The listing builds one solid part. Answer for the finished solid, in the listing's coordinates (mm). A direction names the side the tool comes from. Coordinates: 2 decimals unless noted, no trailing zeros. Order: outer loops, then holes, each group sorted by start corner. A loop starts at its lowest first (then second) coordinate and runs counter-clockwise, first axis right, second up. Notation, with made-up numbers: (47, 76) -> (86, 76) arc R28 ccw to (86, 99) -> close; hole circle Ø9 at (-13, 12.25). An arc over 180 degrees is marked (long way). Return JSON: item names as keys, results as strings.
from build123d import *

# Parameters (mm, degrees)
SKETCH1_R               = 5.15
BOSS_EXTRUDE1_DEPTH     = 10.3
SKETCH2_R               = 1
CUT_EXTRUDE1_DEPTH      = 10
CUT_EXTRUDE1_DEPTH_BACK = 10
SKETCH3_W               = 4.05
SKETCH3_H               = 4.05
CUT_EXTRUDE2_DEPTH      = 5


with BuildPart() as part:
    # Sketch1 → Boss-Extrude1 (new body)
    with BuildSketch(Plane.XY):
        Circle(SKETCH1_R)
    extrude(amount=BOSS_EXTRUDE1_DEPTH)

    # Sketch2 → Cut-Extrude1 (cut, two sides)
    with BuildSketch(Plane(origin=(0, 0, 0), x_dir=(1, 0, 0), z_dir=(0, 1, 0))) as cut_extrude1_sk:
        with Locations((0, -7.5)):
            Circle(SKETCH2_R)
    extrude(amount=CUT_EXTRUDE1_DEPTH, mode=Mode.SUBTRACT)
    extrude(cut_extrude1_sk.sketch, amount=-CUT_EXTRUDE1_DEPTH_BACK, mode=Mode.SUBTRACT)

    # Sketch3 → Cut-Extrude2 (cut)
    with BuildSketch(Plane(origin=(0, 0, 0), x_dir=(-1, 0, 0), z_dir=(0, 0, -1))):
        Rectangle(SKETCH3_W, SKETCH3_H)
    extrude(amount=-CUT_EXTRUDE2_DEPTH, mode=Mode.SUBTRACT)


solid = part.part
1. The part is cut by section A-A on x = 0. Give the vertices of the cut face in (y, z) (3 decimals), and give its area (3 significant figures).
Answer block:
{"outline": "(-5.15, 0) -> (-2.025, 0) -> (-2.025, 5) -> (2.025, 5) -> (2.025, 0) -> (5.15, 0) -> (5.15, 6.5) -> (-5.15, 6.5) -> close; (-5.15, 8.5) -> (5.15, 8.5) -> (5.15, 10.3) -> (-5.15, 10.3) -> close", "area": "65.2 mm2"}
2. The part is cut by section C-C on y = 0.75. Give the vertices of the cut face in (x, z) (3 decimals).
Answer block:
{"outline": "(-5.095, 0) -> (-2.025, 0) -> (-2.025, 5) -> (2.025, 5) -> (2.025, 0) -> (5.095, 0) -> (5.095, 10.3) -> (-5.095, 10.3) -> close; hole circle Ø2 at (0, 7.5)"}
3. Consider line 1 (Z direction, x = 0, y = -3.95); line 2 (Z direction, x = 0, y = 1.65); line 3 (Y direction, x = 0.5, z = 3.5) (3 decimals). Determine where each line is inside the solid, lowest interval first. Write a range as from..to.
Answer block:
{"line 1": "z = 0..6.5, 8.5..10.3", "line 2": "z = 5..6.5, 8.5..10.3", "line 3": "y = -5.126..-2.025, 2.025..5.126"}
4. The part is cut by section D-D on x = 1.25. Give the vertices of the cut face in (y, z) (3 decimals).
Answer block:
{"outline": "(-4.996, 0) -> (-2.025, 0) -> (-2.025, 5) -> (2.025, 5) -> (2.025, 0) -> (4.996, 0) -> (4.996, 10.3) -> (-4.996, 10.3) -> close"}
5. The part is cut by section B-B on z = 4. Give the vertices of the cut face in (x, y) (3 decimals), and give its area (3 significant figures).
Answer block:
{"outline": "circle Ø10.3 at (0, 0); hole (-2.025, -2.025) -> (2.025, -2.025) -> (2.025, 2.025) -> (-2.025, 2.025) -> close", "area": "66.9 mm2"}
6. Each of these flat-tipped pins is pushed along its axis until it touches: pin 1 Ø1 at (y, z) = (-4, 2) entering from +X; pin 2 Ø2 at (x, z) = (-1, 1.5) entering from -Y; pin 3 Ø1.6 at (x, z) = (0, 7.5) entering from +Y; pin 4 Ø6 at (y, z) = (-3.5, 1.5) entering from +X. Where does it stop, or does it pass through?
Answer block:
{"pin 1": "stops at x = 3.78", "pin 2": "stops at y = -5.15", "pin 3": "passes through", "pin 4": "stops at x = 5.13"}
7. For faces 1 (the face through (-0.1, -2.2, 0)), 2 (the face through (-2.025, 0, 2)), determine the directions among +Z, -Z, +X, -X, +Y, -Y from which every point of the face is accessible in a straight line to the end or side of a thin tool.
Answer block:
{"face 1": "-Z, +X, -X, +Y, -Y", "face 2": "-Z"}
8. Determine the mould class of faces 3 (the face through (2.025, 0, 2)), 4 (the face through (0, 0, 10.3)), 5 (the face through (-1.116, -5.028, 5.078)) for opening direction X: pulls with the +X half, pulls with the -X half, needs draft (parallel to the pull), parting line crosses it, or undercut.
Answer block:
{"face 3": "undercut", "face 4": "needs draft", "face 5": "parting line crosses it"}
